Could you check a few things on this model? Use its own coordinates, in mm. Face numbers are marked on the shaded views. A direction names the side the tool comes from. Coordinates: 2 decimals unless noted, no trailing zeros. Loops run counter-clockwise (first coordinate to the right, second up) from the corner with the lowest first, then second, coordinate; pieces in that order, holes last. Notation, with made-up numbers: M -9,41 L 29,41 A14 ccw 29,67 Z; hole C 24.25,35 d6. An arc over 180 degrees is marked long. Write each question's results on one line, items separated by ' | '.
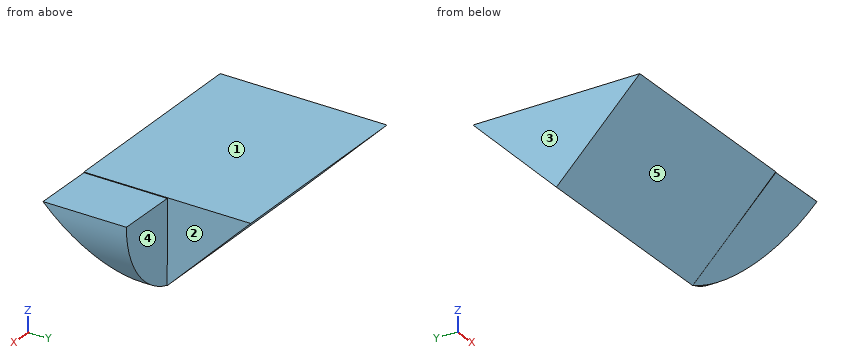
```python
from build123d import *

# Parameters (mm, degrees)
F0_W        = 63.5
F0_H        = 76.2
F1_DEPTH    = 25.4
F2_T1_DEPTH = 259.462243683
F3_T1_DEPTH = 259.462243683
F5_DEPTH    = 25.4
F7_DEPTH    = 25.4


# Not quite as in the source:
# - a fillet or chamfer that OpenCascade refuses, or shapes differently, is made with other operations: its cross-section is extruded or revolved along the edge and cut away or added


with BuildPart() as f1:
    # F0 (on Top) → F1 (new body)
    with BuildSketch(Plane.XY):
        Rectangle(F0_W, F0_H)
    extrude(amount=-F1_DEPTH)

    # F2: chamfer of 38.1 on 1 edges, made by hand

    # F2_s2 → F2_t1 (cut)
    with BuildSketch(Plane.YZ.offset(-129.7311218415)):
        Polygon((38.1, 12.7), (0, -25.4), (38.1, -25.4), align=None)
    extrude(amount=F2_T1_DEPTH, mode=Mode.SUBTRACT)

    # F3: chamfer of 38.1 on 1 edges, made by hand

    # F3_s2 → F3_t1 (cut)
    with BuildSketch(Plane.YZ.offset(-129.7311218415)):
        Polygon((0, -25.4), (-38.1, 12.7), (-38.1, -25.4), align=None)
    extrude(amount=F3_T1_DEPTH, mode=Mode.SUBTRACT)

    # F4 (on Front) → F5 (join)
    with BuildSketch(Plane.XZ):
        with BuildLine():
            Line((31.6233746707, -0.1989824377), (31.8418294191, -25.3204219043))
            ThreePointArc((31.8418294191, -25.3204219043), (45.6070605547, -15.863879172), (50.8267469704, 0))
            Line((50.8267469704, 0), (31.6233746707, -0.1989824377))
        make_face()
    extrude(amount=F5_DEPTH)

    # F6 (on face) → F7 (cut)
    with BuildSketch(Plane(origin=(31.6192532968, 0, 0.274959404), x_dir=(0, -1, 0), z_dir=(-0.9999621924, 0, -0.0086956199))):
        Polygon((25.4, -0.473959761), (0, -25.5963490453), (25.4, -25.5963490453), align=None)
    extrude(amount=-F7_DEPTH, mode=Mode.SUBTRACT)


solid = f1.part
```
(1) Which directions (+Z, -Z, +X, -X, +Y, -Y) give clear straight access to the entire face, cutting with the end or side of a thin tool? Please do the marked faces 4 and 5.
Reported:
face 4: +Z, -Z, +X, +Y | face 5: -Z, -X, -Y
(2) Imagine slicing it at B-B, the plane y = -15. List the corners of the cut face in (x, z) for me.
Reported:
outline: M -31.75,-10.4 L 31.71,-10.4 L 31.71,-10.48 L 48.78,-10.34 A26.11 ccw 50.83,0 L 31.75,-0.2 L 31.75,0 L -31.75,0 Z
(3) Will these pins go through, and if not, where does the flat tip stop? P1, Ø10, axis at x = -7, z = -19, coming from the -Y side; P2, Ø8, axis at x = 38, z = -13.5, coming from the +Y side; P3, Ø10, axis at y = -9, z = -20, coming from the +X side.
Reported:
P1: stops at y = -11.4 | P2: stops at y = 0 | P3: stops at x = 46.23
(4) If we mould it in two halves opening along X, with no side actions, what happens to the marked faces 1, 2 and 3? For each: released by +X, released by -X, zero draft, split by the parting line, or undercut.
Reported:
face 1: zero draft | face 2: undercut | face 3: released by -X
(5) Imagine slicing it at A-A, the plane z = -16.25. List the corners of the cut face in (x, y) for me.
Reported:
outline: M -31.75,-9.15 L 31.75,-9.15 L 31.75,9.15 L -31.75,9.15 Z; M 31.76,-9.17 L 45.31,-9.05 L 45.31,0 L 31.76,0 Z
(6) Imagine slicing it at C-C, the plane z = -8. List the corners of the cut face in (x, y) for me, and give its area (3 significant figures).
Reported:
outline: M -31.75,-17.4 L 31.69,-17.4 L 31.69,-17.51 L 49.64,-17.35 L 49.64,0 L 31.75,0 L 31.75,17.4 L -31.75,17.4 Z | area: 2,520 mm2
(7) Please list where these lines run through material, in increasing order: probe 1 along X at (y, z) = (22, -1.75); probe 2 along Y at (x, z) = (-18, -2); probe 3 along Z at (x, y) = (-18.5, 13). Write a range as from..to.
Reported:
probe 1: x = -31.75..31.75 | probe 2: y = -23.4..23.4 | probe 3: z = -12.4..0
(8) Imagine slicing it at D-D, the plane z = -23.5. List the corners of the cut face in (x, y) for me.
Reported:
outline: M -31.75,-1.9 L 31.75,-1.9 L 31.75,1.9 L -31.75,1.9 Z; M 31.83,-1.84 L 36.5,-1.8 L 36.5,0 L 31.83,0 Z
